Can you work these out from the drawing? Everything is in mm from the part's minimum corner. A direction names the side the tool comes from. Coordinates: 2 decimals unless noted, no trailing zeros. Order: outer loops, then holes, each group sorted by start corner. A loop starts at its lowest first (then second) coordinate and runs counter-clockwise, first axis right, second up. Notation, with made-up numbers: (-15.5, -2) -> (1.5, -2) arc R24 ccw to (1.5, 23) -> close; hole circle Ø11 at (-30.5, 66). An arc over 180 degrees is marked (long way). Answer in a Markdown table with one row per item.
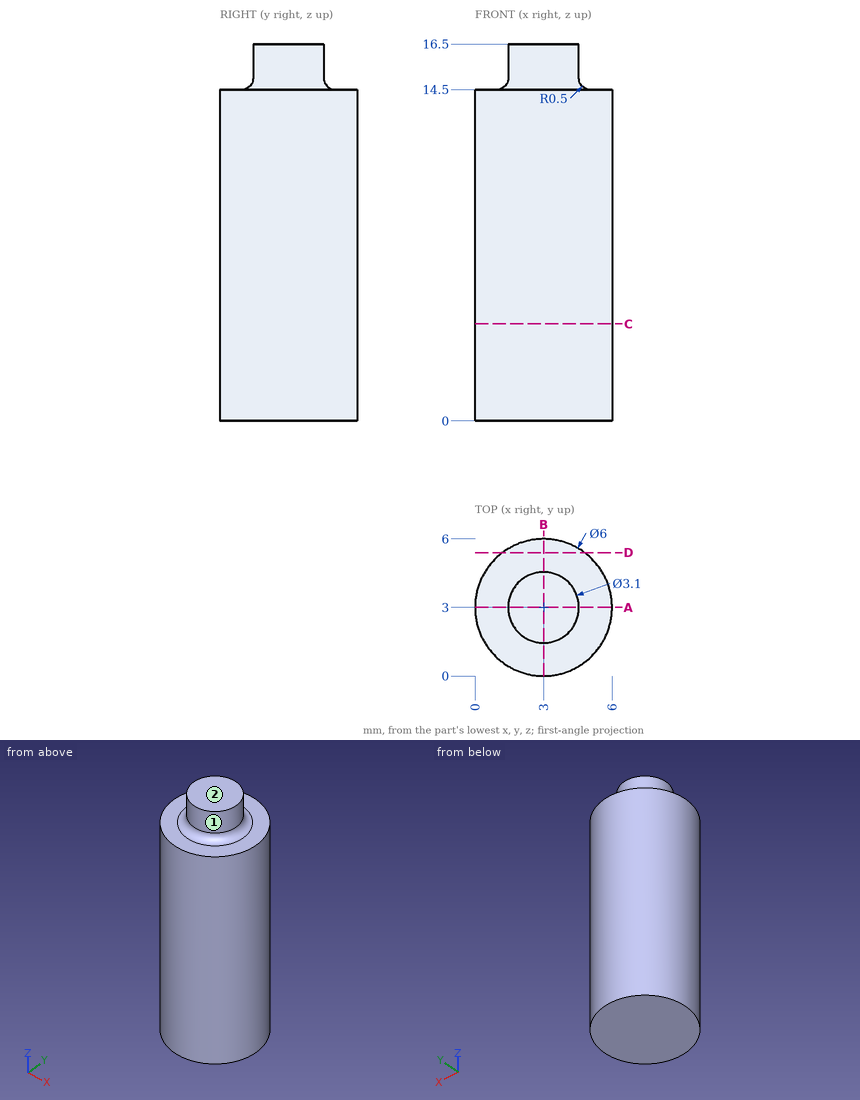
(1) Suppose I cut it at A-A (y = 3). Please give me the cut outline in (x, z).
Response values:
| item | result |
|---|---|
| outline | (0, 0) -> (6, 0) -> (6, 14.5) -> (5.05, 14.5) arc R0.5 cw to (4.55, 15) -> (4.55, 16.5) -> (1.45, 16.5) -> (1.45, 15) arc R0.5 cw to (0.95, 14.5) -> (0, 14.5) -> close |
(2) Suppose I cut it at C-C (z = 4.25). Please give me the cut outline in (x, y), and give its area (3 significant figures).
Response values:
| item | result |
|---|---|
| outline | circle Ø6 at (3, 3) |
| area | 28.3 mm2 |
(3) Suppose I cut it at D-D (y = 5.4). Please give me the cut outline in (x, z), and give its area (3 significant figures).
Response values:
| item | result |
|---|---|
| outline | (1.2, 0) -> (4.8, 0) -> (4.8, 14.5) -> (1.2, 14.5) -> close |
| area | 52.2 mm2 |
(4) I need wall thicknesses on line 1 (Z direction, x = 4.4, y = 1.4); line 2 (Y direction, x = 2.45, z = 3.75); line 3 (X direction, y = 2.3, z = 1.75). Which ranges of each line are inside material? Lowest first, please. Write a range as [from, to].
Response values:
| item | result |
|---|---|
| line 1 | [0, 14.5] |
| line 2 | [0.05, 5.95] |
| line 3 | [0.08, 5.92] |
(5) On a 3-axis mill with a long thin cutter (end or side, diameter ignored), from which of +Z, -Z, +X, -X, +Y, -Y can I reach the whole of each face in a straight line? I mean the marked faces 1 and 2. Say none if no direction works.
Response values:
| item | result |
|---|---|
| face 1 | +Z |
| face 2 | +Z, +X, -X, +Y, -Y |
